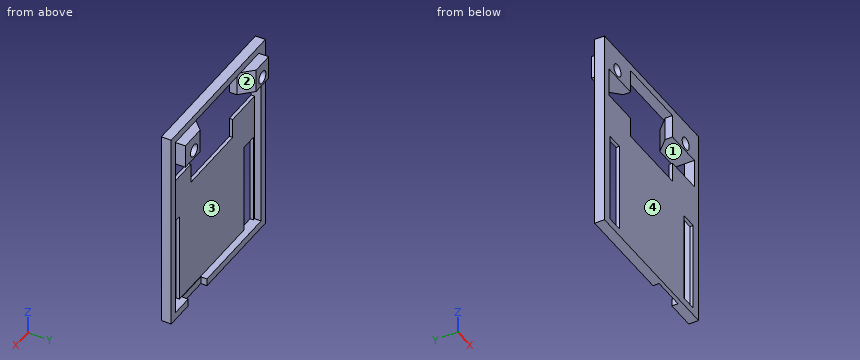
```python
from build123d import *

# Parameters (mm, degrees)
SKETCH1_W           = 40
SKETCH1_H           = 49
BOSS_EXTRUDE1_DEPTH = 2.4
SKETCH2_W           = 36.4
SKETCH2_H           = 45.4
CUT_EXTRUDE1_DEPTH  = 1.6
SKETCH3_W           = 9.3
SKETCH3_H           = 7
SKETCH3_W_2         = 4
SKETCH3_H_2         = 22
CUT_EXTRUDE2_DEPTH  = 1.6
SKETCH4_W           = 9.3
SKETCH4_H           = 5.7
BOSS_EXTRUDE2_DEPTH = 4
SKETCH5_R           = 1.5
CUT_EXTRUDE3_DEPTH  = 5
CHAMFER1_SIZE       = 3
SKETCH6_W           = 8
SKETCH6_H           = 1.8
CUT_EXTRUDE4_DEPTH  = 1.5
SKETCH7_W           = 1
SKETCH7_H           = 5.7
CUT_EXTRUDE5_DEPTH  = 2.4


with BuildPart() as part:
    # Sketch1 → Boss-Extrude1 (new body)
    with BuildSketch(Plane(origin=(0, 0, 0), x_dir=(1, 0, 0), z_dir=(0, 1, 0))):
        Rectangle(SKETCH1_W, SKETCH1_H)
    extrude(amount=BOSS_EXTRUDE1_DEPTH)

    # Sketch2 → Cut-Extrude1 (cut)
    with BuildSketch(Plane(origin=(0, 2.4, 0), x_dir=(1, 0, 0), z_dir=(0, 1, 0))):
        Rectangle(SKETCH2_W, SKETCH2_H)
    extrude(amount=-CUT_EXTRUDE1_DEPTH, mode=Mode.SUBTRACT)

    # Sketch3 → Cut-Extrude2 (cut)
    with BuildSketch(Plane(origin=(0, 0.8, 0), x_dir=(1, 0, 0), z_dir=(0, 1, 0))):
        with Locations((-13.55, -13.5)):
            Rectangle(SKETCH3_W, SKETCH3_H)
        Polygon((8.9, -5.2), (-8.9, -5.2), (-8.9, -10), (-8.9, -17), (-8.9, -22.7), (8.9, -22.7), (8.9, -17), (8.9, -10), align=None)
        with Locations((13.55, -13.5)):
            Rectangle(SKETCH3_W, SKETCH3_H)
        with Locations((15.7, 11.7)):
            Rectangle(SKETCH3_W_2, SKETCH3_H_2)
        with Locations((-15.7, 11.7)):
            Rectangle(SKETCH3_W_2, SKETCH3_H_2)
    extrude(amount=-CUT_EXTRUDE2_DEPTH, mode=Mode.SUBTRACT)

    # Sketch4 → Boss-Extrude2 (add)
    with BuildSketch(Plane(origin=(0, 0.8, 0), x_dir=(1, 0, 0), z_dir=(0, 1, 0))):
        with Locations((-13.55, -19.85)):
            Rectangle(SKETCH4_W, SKETCH4_H)
        with Locations((13.55, -19.85)):
            Rectangle(SKETCH4_W, SKETCH4_H)
    extrude(amount=BOSS_EXTRUDE2_DEPTH)

    # Sketch5 → Cut-Extrude3 (cut)
    with BuildSketch(Plane(origin=(0, 4.8, 0), x_dir=(1, 0, 0), z_dir=(0, 1, 0))):
        with Locations(Location((-14.5, -19, 0), (0, 0, 270))):
            Circle(SKETCH5_R)
        with Locations(Location((14.5, -19, 0), (0, 0, 270))):
            Circle(SKETCH5_R)
    extrude(amount=-CUT_EXTRUDE3_DEPTH, mode=Mode.SUBTRACT)

    # Chamfer1
    # the kernel refuses this chamfer: 3 mm, written as the material it takes off along each edge
    with BuildSketch(Plane(origin=(-8.9, 4.8, 22.7), x_dir=(0.02749587661058793, -0.9996219169112968, 0), z_dir=(0, 0, -1)), Plane(origin=(8.9, 4.8, 9.284951036), x_dir=(-0.027495876610586202, -0.9996219169112968, 0), z_dir=(0, 0, 1))) as chamfer1_piece_1:
        Polygon((CHAMFER1_SIZE * 0.999621916911, CHAMFER1_SIZE * 0.0274958766106), (-CHAMFER1_SIZE * 0.0274958766106, CHAMFER1_SIZE * 0.999621916911), (0, 0), align=None)
    extrude(amount=13.415048964, mode=Mode.SUBTRACT)

    # Sketch6 → Cut-Extrude4 (cut)
    with BuildSketch(Plane(origin=(0, 2.4, 0), x_dir=(1, 0, 0), z_dir=(0, 1, 0))):
        with Locations((8.8, 23.6)):
            Rectangle(SKETCH6_W, SKETCH6_H)
    extrude(amount=-CUT_EXTRUDE4_DEPTH, mode=Mode.SUBTRACT)

    # Sketch7 → Cut-Extrude5 (cut)
    with BuildSketch(Plane(origin=(0, 4.8, 0), x_dir=(1, 0, 0), z_dir=(0, 1, 0))):
        with Locations((-17.7, -19.85)):
            Rectangle(SKETCH7_W, SKETCH7_H)
    extrude(amount=-CUT_EXTRUDE5_DEPTH, mode=Mode.SUBTRACT)


solid = part.part
```
Read the model definition and answer for the solid it produces. Units are mm, in the model's axes. Face numbers are marked on the shaded views. A direction names the side the tool comes from. Coordinates: 2 decimals unless noted, no trailing zeros. Loops run counter-clockwise (first coordinate to the right, second up) from the corner with the lowest first, then second, coordinate; pieces in that order, holes last. Notation, with made-up numbers: (-13.5, 45.5) -> (27.5, 45.5) arc R8 ccw to (27.5, 57.5) -> close; hole circle Ø4 at (31, 62.5). An arc over 180 degrees is marked (long way). Return JSON: item names as keys, results as strings.
Item 1: Flat-ended cylindrical pins translate along their axes: P1, Ø6, axis at x = 0, z = 10, coming from the -Y side; P2, Ø3, axis at x = 4.5, z = 2.5, coming from the -Y side; P3, Ø1.2, axis at y = 4, z = 19, coming from the -X side; P4, Ø1.4, axis at x = 9, z = -24, coming from the +Y side. Find the tip coordinate at first contact, or state that the pin passes through.
Answers:
{"P1": "passes through", "P2": "stops at y = 0", "P3": "stops at x = -17.2", "P4": "stops at y = 0.9"}
Item 2: Find the intervals of material crossed by probe 1 along X at (y, z) = (0.65, -9); probe 2 along X at (y, z) = (1.3, -16.5); probe 3 along X at (y, z) = (1.2, 21.5), in increasing order.
Answers:
{"probe 1": "x = -20 to -17.7, -13.7 to 13.7, 17.7 to 20", "probe 2": "x = -20 to -18.2, 18.2 to 20", "probe 3": "x = -20 to -8.9, 8.9 to 20"}
Item 3: For a pull along X with two mould halves and no side action, classify the marked faces 3 and 4 as +X half, -X half, draft (parallel to the pull), parting line (faces both ways), or undercut.
Answers:
{"face 3": "undercut", "face 4": "draft"}
Item 4: For the marked faces 1 and 2, determine the directions among +Z, -Z, +X, -X, +Y, -Y from which every point of the face is accessible in a straight line to the end or side of a thin tool.
Answers:
{"face 1": "+Y, -Y", "face 2": "+Y"}
Item 5: Find section B-B (z = 19). Determine the outline of the cut face in (x, y), plus the area to 3 significant figures.
Answers:
{"outline": "(-20, 0) -> (-16, 0) -> (-16, 4.8) -> (-17.2, 4.8) -> (-17.2, 2.4) -> (-20, 2.4) -> close; (-13, 0) -> (-8.9, 0) -> (-8.9, 1.8) -> (-11.9, 4.8) -> (-13, 4.8) -> close; (8.9, 0) -> (13, 0) -> (13, 4.8) -> (11.9, 4.8) -> (8.9, 1.8) -> close; (16, 0) -> (20, 0) -> (20, 2.4) -> (18.2, 2.4) -> (18.2, 4.8) -> (16, 4.8) -> close", "area": "57.7 mm2"}
Item 6: Find section D-D (x = -7). Determine the outline of the cut face in (y, z), plus the area to 3 significant figures.
Answers:
{"outline": "(0, -24.5) -> (2.4, -24.5) -> (2.4, -22.7) -> (0.8, -22.7) -> (0.8, 5.2) -> (0, 5.2) -> close; (0, 22.7) -> (2.4, 22.7) -> (2.4, 24.5) -> (0, 24.5) -> close", "area": "31.0 mm2"}
Item 7: Find section C-C (x = 17). Determine the outline of the cut face in (y, z).
Answers:
{"outline": "(0, -24.5) -> (2.4, -24.5) -> (2.4, -22.7) -> (0, -22.7) -> close; (0, -0.7) -> (0.8, -0.7) -> (0.8, 10) -> (0, 10) -> close; (0, 17) -> (4.8, 17) -> (4.8, 22.7) -> (2.4, 22.7) -> (2.4, 24.5) -> (0, 24.5) -> close"}
Item 8: Find section A-A (y = 3.4). Determine the outline of the cut face in (x, z), plus the area to 3 significant figures.
Answers:
{"outline": "(-17.2, 17) -> (-10.5, 17) -> (-10.5, 22.7) -> (-17.2, 22.7) -> close; (10.5, 17) -> (18.2, 17) -> (18.2, 22.7) -> (10.5, 22.7) -> close; hole circle Ø3 at (-14.5, 19); hole circle Ø3 at (14.5, 19)", "area": "67.9 mm2"}
